from build123d import *

# Parameters (mm, degrees)
SKETCH1_W           = 314.43168
SKETCH1_H           = 3.175
BOSS_EXTRUDE1_DEPTH = 200.66180012
CUT_EXTRUDE2_START  = -3.175
SKETCH5_W           = 3.175
SKETCH5_H           = 41.275
CUT_EXTRUDE2_DEPTH  = 259.11040162
BOSS_EXTRUDE3_DEPTH = 3.175
SKETCH12_W          = 101.6
SKETCH12_H          = 3.175
BOSS_EXTRUDE5_DEPTH = 3.175


with BuildPart() as part:
    # Sketch1 → Boss-Extrude1 (new body)
    with BuildSketch(Plane.XY):
        Rectangle(SKETCH1_W, SKETCH1_H)
    extrude(amount=BOSS_EXTRUDE1_DEPTH)

    # Sketch5 → Cut-Extrude2 (cut)
    with BuildSketch(Plane(origin=(0, 1.5875, 0), x_dir=(1, 0, 0), z_dir=(0, 1, 0)).offset(CUT_EXTRUDE2_START)):
        with Locations((-155.62834, -180.02430012)):
            Rectangle(SKETCH5_W, SKETCH5_H)
    cut_extrude2 = extrude(amount=CUT_EXTRUDE2_DEPTH, mode=Mode.SUBTRACT)

    # Mirror1: Cut-Extrude2 across plane
    add(cut_extrude2.mirror(Plane(origin=(0, 0, 0), x_dir=(0, 0, 1), z_dir=(1, 0, 0))), mode=Mode.SUBTRACT)

    # Sketch10 → Boss-Extrude3 (add)
    with BuildSketch(Plane.XZ.offset(1.5875)):
        Polygon((201.6506, 0), (201.6506, 3.175), (160.39084, 50.8), (157.21584, 50.8), (157.21584, 0), align=None)
    extrude(amount=-BOSS_EXTRUDE3_DEPTH)

    # Sketch12 → Boss-Extrude5 (add)
    with BuildSketch(Plane(origin=(0, 0, 0), x_dir=(-1, 0, 0), z_dir=(0, 0, -1))):
        with Locations((-77.02050001, 0)):
            Rectangle(SKETCH12_W, SKETCH12_H)
    boss_extrude5 = extrude(amount=BOSS_EXTRUDE5_DEPTH)

    # Mirror2: Boss-Extrude5 across plane
    add(boss_extrude5.mirror(Plane(origin=(0, 0, 0), x_dir=(0, 0, 1), z_dir=(1, 0, 0))))


solid = part.part
The listing builds one solid part. Answer for the finished solid, in the listing's coordinates (mm). Coordinates: 2 decimals unless noted, no trailing zeros. Write each loop counter-clockwise with the first axis right and the second up, starting at its lowest first coordinate (ties: lowest second). Pieces come first, ordered by that corner, then holes. Notation, with made-up numbers: (50.25, -20.5) -> (58.25, -20.5) arc R17 ccw to (58.25, -6.5) -> close; hole circle Ø7 at (44, 89). An arc over 180 degrees is marked (long way). One line per question, with ' | ' between items.
1. Straight lines are drawn through the part: line 1 (Z direction, x = -8, y = 0.95); line 2 (X direction, y = 0.6, z = 60); line 3 (X direction, y = -1.25, z = 186.5). For each, find the intervals that lie inside material, in ascending order.
Verdict:
line 1: z = 0 to 200.66 | line 2: x = -157.22 to 157.22 | line 3: x = -154.04 to 154.04
2. Section B-B (z = 182) is taken. Determine the outline of the cut face in (x, y).
Verdict:
outline: (-154.04, -1.59) -> (154.04, -1.59) -> (154.04, 1.59) -> (-154.04, 1.59) -> close
3. Section A-A (y = -0.15) is taken. Determine the outline of the cut face in (x, z) (1 decimal), and give its area (3 significant figures).
Verdict:
outline: (-157.2, 0) -> (-127.8, 0) -> (-127.8, -3.2) -> (-26.2, -3.2) -> (-26.2, 0) -> (26.2, 0) -> (26.2, -3.2) -> (127.8, -3.2) -> (127.8, 0) -> (201.7, 0) -> (201.7, 3.2) -> (160.4, 50.8) -> (157.2, 50.8) -> (157.2, 159.4) -> (154, 159.4) -> (154, 200.7) -> (-154, 200.7) -> (-154, 159.4) -> (-157.2, 159.4) -> close | area: 64,800 mm^2
4. Given pin 1 Ø1.6 at (x, y) = (176.5, -0.5) entering from -Z; pin 2 Ø1.6 at (y, z) = (-0.5, 89.5) entering from +X; pin 3 Ø1.6 at (y, z) = (0.5, 180.5) entering from +X, each flat-ended and moving along its own axis, determine where each tip first touches the part or whether it passes through.
Verdict:
pin 1: stops at z = 0 | pin 2: stops at x = 157.22 | pin 3: stops at x = 154.04
5. Section C-C (x = 16.5) is taken. Determine the outline of the cut face in (y, z).
Verdict:
outline: (-1.59, 0) -> (1.59, 0) -> (1.59, 200.66) -> (-1.59, 200.66) -> close
